Geometry: final body of the model. Coordinates: model frame, mm. Face numbers are marked on the shaded views. A direction names the side the tool comes from. Coordinates: 2 decimals unless noted, no trailing zeros. Loops run counter-clockwise (first coordinate to the right, second up) from the corner with the lowest first, then second, coordinate; pieces in that order, holes last. Notation, with made-up numbers: (88.25, -40) - (92.25, -40) arc R7 cw to (92.25, -28) - close; hole circle Ø9 at (16, 41.5). An arc over 180 degrees is marked (long way). Write each question's results on one line, items separated by ' | '. Start each with the question number.
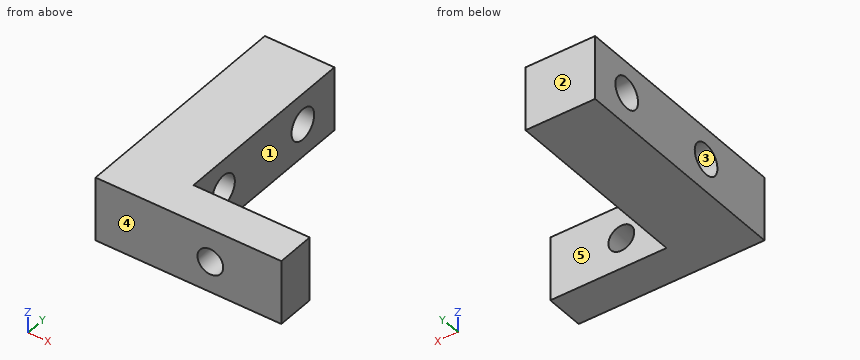
from build123d import *

# Parameters (mm, degrees)
SKETCH1_W           = 18.325664351
SKETCH1_H           = 6.332689346
SKETCH1_R           = 1.27
BOSS_EXTRUDE1_DEPTH = 3.81
SKETCH2_W           = 6.332689346
SKETCH2_H           = 18.949374656
SKETCH2_R           = 1.524
BOSS_EXTRUDE2_DEPTH = 6.864742327


with BuildPart() as part:
    # Sketch1 → Boss-Extrude1 (new body)
    with BuildSketch(Plane(origin=(0, 0, 0), x_dir=(1, 0, 0), z_dir=(0, 1, 0))):
        with Locations((9.162832176, 3.166344673)):
            Rectangle(SKETCH1_W, SKETCH1_H)
        with Locations(Location((11.320424566, 3.284411685, 0), (0, 0, 90))):
            Circle(SKETCH1_R, mode=Mode.SUBTRACT)
    extrude(amount=BOSS_EXTRUDE1_DEPTH)

    # Sketch2 → Boss-Extrude2 (add)
    with BuildSketch(Plane.ZY):
        with Locations((-3.166344673, 13.284687328)):
            Rectangle(SKETCH2_W, SKETCH2_H)
        with Locations((-3.080246652, 18.514377614)):
            Circle(SKETCH2_R, mode=Mode.SUBTRACT)
        with Locations((-3.080246652, 7.846377614)):
            Circle(SKETCH2_R, mode=Mode.SUBTRACT)
    extrude(amount=-BOSS_EXTRUDE2_DEPTH)


solid = part.part
1) Pin query (flat end, axial travel): pin 1 Ø1.8 at (y, z) = (7.85, -3.08) entering from +X; pin 2 Ø3 at (x, z) = (12.5, -4) entering from +Y. Return the tip coordinate at first contact, or that it passes through.
2) Section query A-A on z = -2.75. Output: boundary loops of the cut face in (x, y).
3) Section query D-D on x = 2.5. Output: boundary loops of the cut face in (y, z), and give its area (3 significant figures).
4) Pull-direction query (Y, two-part tool) for the marked faces 3, 4 and 5; classes: released by +Y, released by -Y, zero draft, split by the parting line, or undercut.
5) Material intervals for line 1 (Z direction, x = 3, y = 18.5); line 2 (Y direction, x = 2.25, z = -3.75); line 3 (Y direction, x = 4, z = -4.25), sorted ascending. Write a range as [from, to].
6) Access query for the marked faces 1 and 2. Directions: +Z, -Z, +X, -X, +Y, -Y. A direction counts if a zero-diameter tool reaches every point of the face in a straight line with its end or side. Return the directions, or none.
7) Section query C-C on y = 1.5. Output: boundary loops of the cut face in (x, z).
8) Section query B-B on y = 6.75. Output: boundary loops of the cut face in (x, z), and give its area (3 significant figures).
Returned:
1) pin 1: passes through | pin 2: stops at y = 3.81
2) outline: (0, 0) - (10.17, 0) - (10.17, 3.81) - (6.86, 3.81) - (6.86, 6.36) - (0, 6.36) - close; (0, 9.33) - (6.86, 9.33) - (6.86, 17.03) - (0, 17.03) - close; (0, 20) - (6.86, 20) - (6.86, 22.76) - (0, 22.76) - close; (12.47, 0) - (18.33, 0) - (18.33, 3.81) - (12.47, 3.81) - close
3) outline: (0, -6.33) - (22.76, -6.33) - (22.76, 0) - (0, 0) - close; hole circle Ø3.05 at (7.85, -3.08); hole circle Ø3.05 at (18.51, -3.08) | area: 130 mm²
4) face 3: undercut | face 4: released by -Y | face 5: released by +Y
5) line 1: z = [-6.33, -4.6], [-1.56, 0] | line 2: y = [0, 6.48], [9.22, 17.15], [19.88, 22.76] | line 3: y = [0, 6.87], [8.82, 17.54], [19.49, 22.76]
6) face 1: +Z, -Z, +X, +Y | face 2: +Z, -Z, +X, -X, +Y
7) outline: (0, -6.33) - (18.33, -6.33) - (18.33, 0) - (0, 0) - close; hole circle Ø2.54 at (11.32, -3.28)
8) outline: (0, -6.33) - (6.86, -6.33) - (6.86, -4.14) - (0, -4.14) - close; (0, -2.02) - (6.86, -2.02) - (6.86, 0) - (0, 0) - close | area: 28.9 mm²
